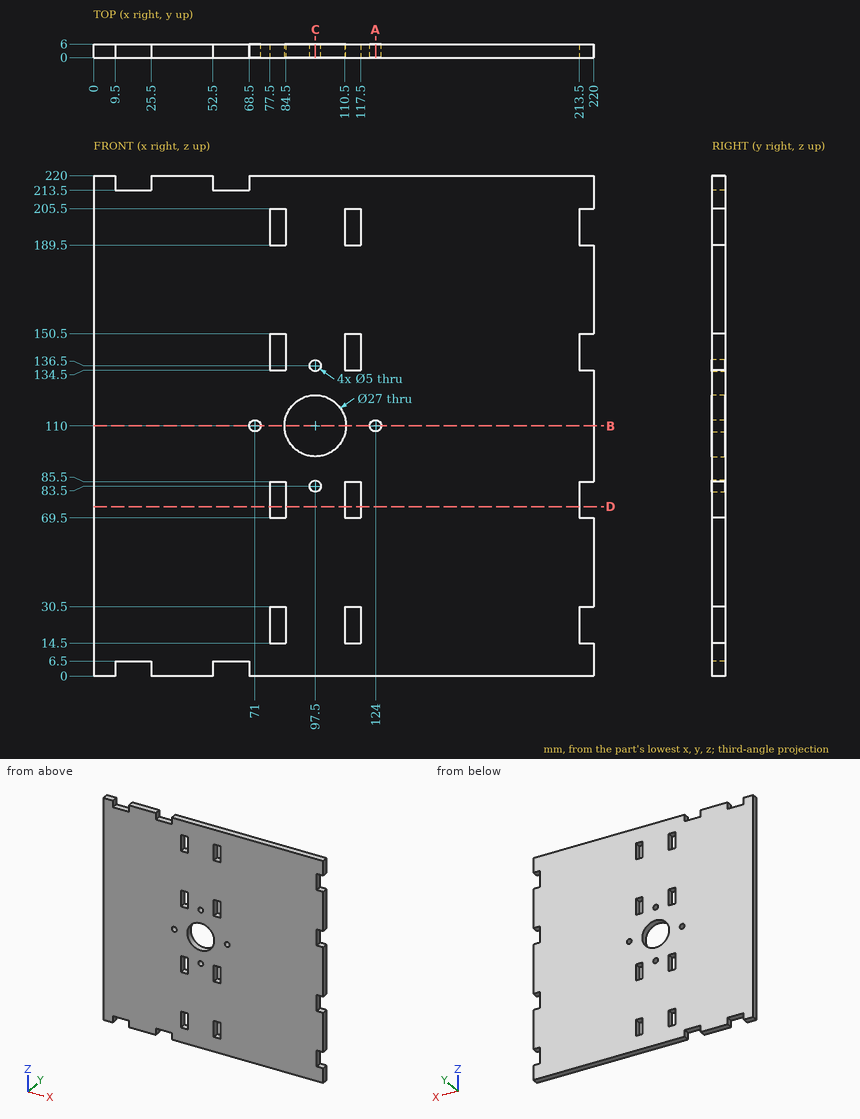
Design review of the part shown in the three views and the two pictorial views. Dimensions are in mm from the part's minimum x, y and z. Give positions to 0.01 mm unless a question says otherwise; leave off trailing zeros. Loops run counter-clockwise (first coordinate to the right, second up) from the corner with the lowest first, then second, coordinate; pieces in that order, holes last. Notation, with made-up numbers: (-18, 62.5) - (29, 62.5) arc R33 cw to (29, 99.5) - close; hole circle Ø11 at (80, -3.75). An arc over 180 degrees is marked (long way). Use CSV: the item, a comma, the result in double quotes. Start each with the question number.
1. Wall thickness on L1, parallel to X at y = 1.4, z = 110; L2, parallel to X at y = 5.45, z = 197; L3, parallel to X at y = 4.55, z = 83.5: over which ranges is each line inside the solid? List them lowest first.
2. Add section A-A (x = 124). State the section outline as (y, z) points, plus the area to 3 significant figures.
3. Add section C-C (x = 97.5). State the section outline as (y, z) points, plus the area to 3 significant figures.
4. Add section B-B (z = 110). State the section outline as (x, y) points, plus the area to 3 significant figures.
5. Add section D-D (z = 74.5). State the section outline as (x, y) points.
Results found:
1,L1,"x = 0 to 68.5, 73.5 to 84, 111 to 121.5, 126.5 to 220"
1,L2,"x = 0 to 77.5, 84.5 to 110.5, 117.5 to 213.5"
1,L3,"x = 0 to 77.5, 84.5 to 95, 100 to 110.5, 117.5 to 213.5"
2,outline,"(0, 0) - (6, 0) - (6, 107.5) - (0, 107.5) - close; (0, 112.5) - (6, 112.5) - (6, 220) - (0, 220) - close"
2,area,"1,290 mm²"
3,outline,"(0, 0) - (6, 0) - (6, 81) - (0, 81) - close; (0, 86) - (6, 86) - (6, 96.5) - (0, 96.5) - close; (0, 123.5) - (6, 123.5) - (6, 134) - (0, 134) - close; (0, 139) - (6, 139) - (6, 220) - (0, 220) - close"
3,area,"1,100 mm²"
4,outline,"(0, 0) - (68.5, 0) - (68.5, 6) - (0, 6) - close; (73.5, 0) - (84, 0) - (84, 6) - (73.5, 6) - close; (111, 0) - (121.5, 0) - (121.5, 6) - (111, 6) - close; (126.5, 0) - (220, 0) - (220, 6) - (126.5, 6) - close"
4,area,"1,100 mm²"
5,outline,"(0, 0) - (77.5, 0) - (77.5, 6) - (0, 6) - close; (84.5, 0) - (110.5, 0) - (110.5, 6) - (84.5, 6) - close; (117.5, 0) - (213.5, 0) - (213.5, 6) - (117.5, 6) - close"
